from build123d import *

# Parameters (mm, degrees)
SKETCH_1_W      = 18
SKETCH_1_H      = 20
EXTRUDE_1_DEPTH = 3
SKETCH_2_W      = 18
SKETCH_2_H      = 3
EXTRUDE_2_DEPTH = 17
HOLE_WIZARD_1_D = 5.5
HOLE_WIZARD_2_D = 5.5
FILLET_1_R      = 2


with BuildPart() as part:
    # 草图1 → 凸台-拉伸1 (new body)
    with BuildSketch(Plane(origin=(0, 0, 0), x_dir=(1, 0, 0), z_dir=(0, 1, 0))):
        with Locations((9, 10)):
            Rectangle(SKETCH_1_W, SKETCH_1_H)
    extrude(amount=EXTRUDE_1_DEPTH)

    # 草图2 → 凸台-拉伸2 (add)
    with BuildSketch(Plane(origin=(0, 3, 0), x_dir=(1, 0, 0), z_dir=(0, 1, 0))):
        with Locations((9, 18.5)):
            Rectangle(SKETCH_2_W, SKETCH_2_H)
    extrude(amount=EXTRUDE_2_DEPTH)

    # 孔1 (through all)
    with Locations(Plane(origin=(0, 0, 0), x_dir=(-1, 0, 0), z_dir=(0, -1, 0))):
        with Locations((-9, 10)):
            Hole(HOLE_WIZARD_1_D / 2)

    # 孔2 (through all)
    with Locations(Plane(origin=(0, 0, -20), x_dir=(-1, 0, 0), z_dir=(0, 0, -1))):
        with Locations((-9, 10)):
            Hole(HOLE_WIZARD_2_D / 2)

    # 圆角1
    fillet_1_edges = [part.edges().sort_by_distance(p)[0] for p in [
        (9, 3, -17),
    ]]
    fillet(fillet_1_edges, radius=FILLET_1_R)


solid = part.part
Geometry check sheet. Reference: the model listing, model coordinates, mm. A direction names the side the tool comes from. Round coordinates to 2 decimals unless told otherwise and drop trailing zeros. Loops run counter-clockwise (first coordinate to the right, second up) from the corner with the lowest first, then second, coordinate; pieces in that order, holes last. Notation, with made-up numbers: (-39.75, -11) -> (-8.75, -11) arc R36 cw to (-8.75, 28) -> close; hole circle Ø3 at (66.5, 13). An arc over 180 degrees is marked (long way). Answer as a JSON object with one key per item and string values. Group by question number.
Item 1: Thickness scan on line 1 along X through (y, z) = (2.25, -10); line 2 along Z through (x, y) = (9, 1.25); line 3 along Y through (x, z) = (15, -6.25). Record the ranges inside material, lowest first.
Item 2: Cross-section at A-A, the plane z = -10. Record the cut outline in (x, y).
Item 3: Cross-section at C-C, the plane x = 9. Record the cut outline in (y, z).
Item 4: Cross-section at B-B, the plane y = 10. Record the cut outline in (x, z).
Item 5: Set-up check for faces 1 (the face through (9, 1, 0)), 2 (the face through (9, 3, -6)): record each of +Z, -Z, +X, -X, +Y, -Y from which the full face is reachable in a straight line by a thin tool's end or side.
Item 6: Cross-section at D-D, the plane z = -18. Record the cut outline in (x, y), plus the area to 3 significant figures.
Item 7: Release check for a two-part mould opening along Y. For faces 3 (the face through (8.642, 12.727, -18.479)), 4 (the face through (0, 2.5, -14.4)), 5 (the face through (9, 20, -19)), 6 (the face through (10.9, 0, -12.4)) record: pulls with the +Y half, pulls with the -Y half, needs draft (parallel to the pull), parting line crosses it, or undercut.
Item 8: Depth check by flat-ended pin: pin 1 Ø6 at (x, y) = (7.5, 15.5) entering from +Z; pin 2 Ø4.5 at (x, z) = (11, -7.5) entering from +Y. Enter the tip coordinate at first touch or a pass-through.
Determined:
{
 "1": {"line 1": "x = 0 to 6.25, 11.75 to 18", "line 2": "z = -20 to -12.75, -7.25 to 0", "line 3": "y = 0 to 3"},
 "2": {"outline": "(0, 0) -> (6.25, 0) -> (6.25, 3) -> (0, 3) -> close; (11.75, 0) -> (18, 0) -> (18, 3) -> (11.75, 3) -> close"},
 "3": {"outline": "(0, -20) -> (7.25, -20) -> (7.25, -17) -> (5, -17) arc R2 cw to (3, -15) -> (3, -12.75) -> (0, -12.75) -> close; (0, -7.25) -> (3, -7.25) -> (3, 0) -> (0, 0) -> close; (12.75, -20) -> (20, -20) -> (20, -17) -> (12.75, -17) -> close"},
 "4": {"outline": "(0, -20) -> (6.25, -20) -> (6.25, -17) -> (0, -17) -> close; (11.75, -20) -> (18, -20) -> (18, -17) -> (11.75, -17) -> close"},
 "5": {"face 1": "+Z, +X, -X, +Y, -Y", "face 2": "+Z, +X, -X, +Y"},
 "6": {"outline": "(0, 0) -> (18, 0) -> (18, 20) -> (0, 20) -> close; hole circle Ø5.5 at (9, 10)", "area": "336 mm²"},
 "7": {"face 3": "undercut", "face 4": "needs draft", "face 5": "pulls with the +Y half", "face 6": "pulls with the -Y half"},
 "8": {"pin 1": "stops at z = -17", "pin 2": "stops at y = 3"}
}
